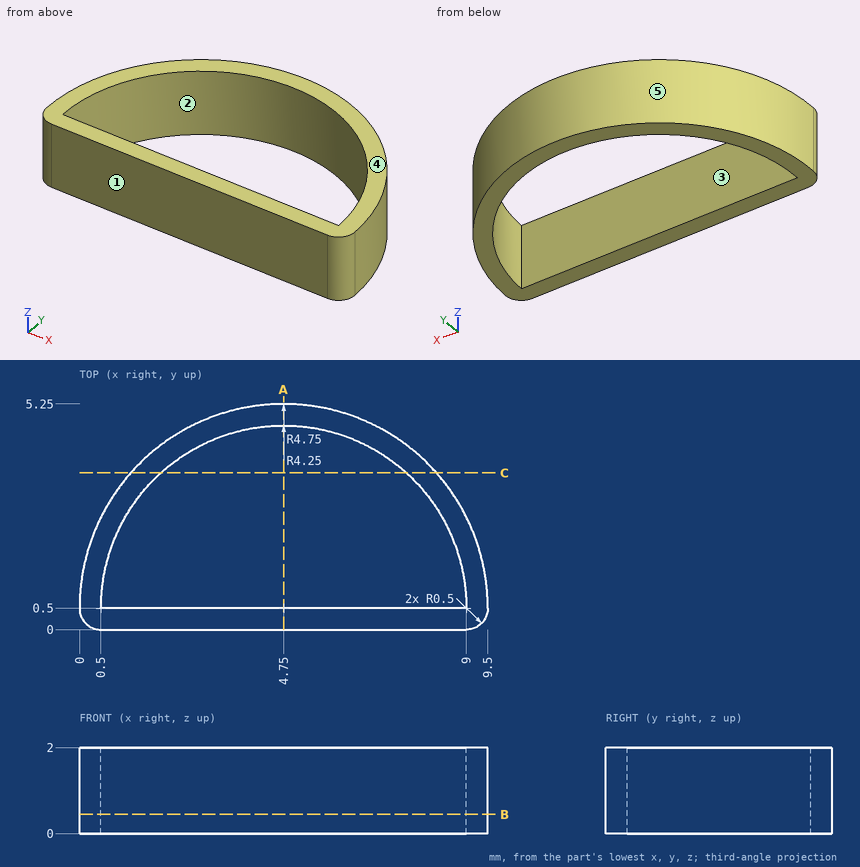
The figure shows three views and two pictorial views of one solid part (mm, origin at its lowest corner). Answer the questions. A direction names the side the tool comes from. Coordinates: 2 decimals unless noted, no trailing zeros. Write each loop counter-clockwise with the first axis right and the second up, starting at its lowest first coordinate (ties: lowest second). Pieces come first, ordered by that corner, then holes. Notation, with made-up numbers: (-1, 15) -> (13, 15) arc R22 ccw to (13, 35) -> close; hole circle Ø1 at (43.25, 71.25). An arc over 180 degrees is marked (long way). Return JSON: item names as keys, results as strings.
(1) For a pull along Y with two mould halves and no side action, classify the marked faces 3, 4 and 5 as pulls with the +Y half, pulls with the -Y half, needs draft (parallel to the pull), parting line crosses it, or undercut.
Answers below:
{"face 3": "undercut", "face 4": "needs draft", "face 5": "pulls with the +Y half"}
(2) Consider line 1 along X through (y, z) = (0.6, 1.1); line 2 along Y through (x, z) = (2, 0.25); line 3 along X through (y, z) = (3.9, 0.6). Determine where each line is inside the solid, lowest interval first. Write a range as from..to.
Answers below:
{"line 1": "0..0.5, 9..9.5", "line 2": "0..0.5, 3.74..4.37", "line 3": "1.43..2.2, 7.3..8.07"}
(3) The part is cut by section A-A on x = 4.75. Give the vertices of the cut face in (y, z), then the cut area to 3 significant figures.
Answers below:
{"outline": "(0, 0) -> (0.5, 0) -> (0.5, 2) -> (0, 2) -> close; (4.75, 0) -> (5.25, 0) -> (5.25, 2) -> (4.75, 2) -> close", "area": "2.00 mm^2"}
(4) Which of the six approach directions +Z, -Z, +X, -X, +Y, -Y give full straight-line access (tool end or side, diameter ignored) to the marked faces 1 and 2?
Answers below:
{"face 1": "+Z, -Z, +X, -X, -Y", "face 2": "+Z, -Z"}
(5) The part is cut by section B-B on z = 0.45. Give the vertices of the cut face in (x, y).
Answers below:
{"outline": "(0, 0.5) arc R0.5 ccw to (0.5, 0) -> (9, 0) arc R0.5 ccw to (9.5, 0.5) arc R4.75 ccw to start; hole (0.5, 0.5) -> (9, 0.5) arc R4.25 ccw to start"}
(6) The part is cut by section C-C on y = 3.65. Give the vertices of the cut face in (x, z), then the cut area to 3 significant figures.
Answers below:
{"outline": "(1.19, 0) -> (1.9, 0) -> (1.9, 2) -> (1.19, 2) -> close; (7.6, 0) -> (8.31, 0) -> (8.31, 2) -> (7.6, 2) -> close", "area": "2.81 mm^2"}
